Autodesk Inventor part; units mm, degrees
ref_plane "YZ Plane" through (0, 0, 0) normal (1, 0, 0) x (0, 1, 0)
ref_plane "XZ Plane" through (0, 0, 0) normal (0, 1, 0) x (-1, 0, 0)
ref_plane "XY Plane" through (0, 0, 0) normal (0, 0, 1) x (1, 0, 0)
sketch "Sketch1" plane through (0, 0, 0) normal (0, 1, 0) x (-1, 0, 0)
  circle A0 centre (0, 0) radius 25.4
  line L0 (0, 25.4) -> (0, 38.1)
  line L1 (0, 0) -> (0, 25.4) construction
  arc A1 (0, 38.1) -> (-25.4, 0) centre (15.875, 0) ccw
  line L2 (0, 0) -> (-25.4, 0) construction
  dimension "d0" = 50.8
  dimension "d1" = 12.7
extrude "Extrusion1" add sketch "Sketch1" along normal blind 96.52
ref_plane "Work Plane1" through (0, 48.26, 0) normal (0, 1, 0) x (1, 0, 0)
sketch "Sketch2" plane through (0, 96.52, 0) normal (0, 1, 0) x (1, 0, 0)
  circle A0 centre (0, -2.54) radius 2.921
  circle A1 centre (0, -2.54) radius 4.7625
  circle A2 centre (0, -2.54) radius 2.286
  point P0 (0, 0)
  dimension "d4" = 2.54
  dimension "d5" = 5.842
  dimension "d6" = 9.525
  dimension "d11" = 4.572
extrude "Extrusion2" add sketch "Sketch2" against normal blind 12.7 from surface at -96.52 contours A0 | A1 | A2
extrude "Extrusion3" cut sketch "Sketch2" against normal blind 13.97 contours A0 | A2
properties part number "Drum"
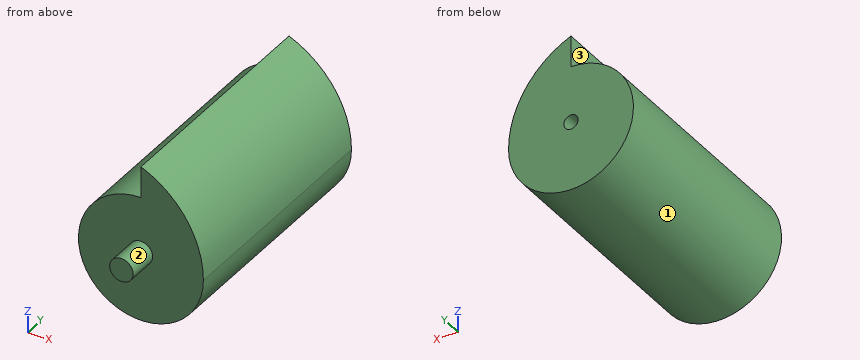
Verification items for the finished model (mm, model axes). Face numbers are marked on the shaded views. A direction names the side the tool comes from. Coordinates: 2 decimals unless noted, no trailing zeros. Write each loop counter-clockwise with the first axis right and the second up, starting at its lowest first coordinate (ties: lowest second). Pieces come first, ordered by that corner, then holes. Notation, with made-up numbers: (81.5, 18) - (124.5, 18) arc R26 cw to (124.5, 33) - close; hole circle Ø11 at (61, 86). An arc over 180 degrees is marked (long way). Answer as a JSON object with one key per item and string values.
(1) Cross-section at C-C on x = -12. Record the cut outline in (y, z), plus the area to 3 significant figures.
Report:
{"outline": "(0, -22.39) - (96.52, -22.39) - (96.52, 22.39) - (0, 22.39) - close", "area": "4,320 mm^2"}
(2) Cross-section at A-A on z = 2.54. Record the cut outline in (x, y).
Report:
{"outline": "(-25.27, 0) - (-4.76, 0) - (-4.76, -12.7) - (4.76, -12.7) - (4.76, 0) - (25.32, 0) - (25.32, 96.52) - (2.92, 96.52) - (2.92, 82.55) - (-2.92, 82.55) - (-2.92, 96.52) - (-25.27, 96.52) - close"}
(3) Tool access check on the marked faces 1, 2 and 3. Record the directions out of +Z, -Z, +X, -X, +Y, -Y that give a thin tool (end or side, any length) a straight path to the whole face; none if there is none.
Report:
{"face 1": "+Y, -Y", "face 2": "-Y", "face 3": "+Z, -X, +Y, -Y"}
(4) Cross-section at B-B on y = 5. Record the cut outline in (x, z) (3 decimals), plus the area to 3 significant figures.
Report:
{"outline": "(0, 25.4) arc R25.4 ccw (long way) to (25.4, 0) arc R41.275 ccw to (0, 38.1) - close", "area": "2,220 mm^2"}
(5) Thickness scan on line 1 along Y through (x, z) = (18, -4.5); line 2 along X through (y, z) = (86, 2); line 3 along X through (y, z) = (87.5, -1). Record the ranges inside material, lowest first.
Report:
{"line 1": "0 to 96.52", "line 2": "-25.32 to -2.87, 2.87 to 25.35", "line 3": "-25.38 to 25.38"}
(6) Gauge pin test, flat ends, axial feed: pin 1 Ø8 at (y, z) = (10, 7.5) entering from -X; pin 2 Ø1.5 at (y, z) = (15, 30.5) entering from -X; pin 3 Ø10 at (x, y) = (-17, 70.5) entering from -Z. Record the tip position at first contact, or that the pin passes through.
Report:
{"pin 1": "x = -25.16", "pin 2": "x = 0", "pin 3": "z = -22.39"}
(7) Cross-section at D-D on x = 7. Record the cut outline in (y, z), plus the area to 3 significant figures.
Report:
{"outline": "(0, -24.42) - (96.52, -24.42) - (96.52, 34.36) - (0, 34.36) - close", "area": "5,670 mm^2"}
